Part model, mm, in its own coordinate system. A direction names the side the tool comes from. Round coordinates to 2 decimals unless told otherwise and drop trailing zeros. Order: outer loops, then holes, each group sorted by start corner. A loop starts at its lowest first (then second) coordinate and runs counter-clockwise, first axis right, second up. Notation, with made-up numbers: (-34.5, 41.5) - (-27.5, 41.5) arc R26 ccw to (-27.5, 66.5) - close; hole circle Ø3 at (64.5, -3.5). An arc over 180 degrees is marked (long way). Answer as a JSON object with one key per item and string values.
```python
from build123d import *

# Parameters (mm, degrees)
RESSALTO_EXTRUS_O1_DEPTH = 6
ESBO_O2_R                = 3.55
RESSALTO_EXTRUS_O2_DEPTH = 2.45
CORTE_EXTRUS_O1_DEPTH    = 12.406502719
CORTE_EXTRUS_O2_REACH    = 13.407
ESBO_O4_R                = 2.525
CHANFRO2_SIZE            = 0.25
CHANFRO3_SIZE            = 0.1


with BuildPart() as part:
    # Esboço1 → Ressalto-extrusão1 (new body)
    with BuildSketch(Plane.XY):
        Polygon((4.961441577, -2.952529562), (5.037686394, 2.820469664), (0.076244817, 5.772999226), (-4.961441577, 2.952529562), (-5.037686394, -2.820469664), (-0.076244817, -5.772999226), align=None)
    extrude(amount=RESSALTO_EXTRUS_O1_DEPTH)

    # Esboço2 → Ressalto-extrusão2 (add)
    with BuildSketch(Plane.XY.offset(6)):
        Circle(ESBO_O2_R)
    extrude(amount=RESSALTO_EXTRUS_O2_DEPTH)

    # Esboço3 → Corte-extrusão1 (cut, through all)
    with BuildSketch(Plane(origin=(0, 0, 0), x_dir=(-1, 0, 0), z_dir=(0, 0, -1))):
        Polygon((-1.65800996, 4.831698543), (-2.173420765, 3.652224278), (-3.376703738, 3.808912301), align=None)
    extrude(amount=-CORTE_EXTRUS_O1_DEPTH, mode=Mode.SUBTRACT)

    # Esboço4 → Corte-extrusão2 (cut, up to next)
    with BuildSketch(Plane.XY.offset(8.45), mode=Mode.PRIVATE) as corte_extrus_o2_sk1:
        with Locations((0, 0.375)):
            Circle(ESBO_O4_R)
    corte_extrus_o2_tool1 = extrude(corte_extrus_o2_sk1.sketch, amount=-CORTE_EXTRUS_O2_REACH, mode=Mode.PRIVATE) & part.part
    add(corte_extrus_o2_tool1.solids().sort_by_distance((0, 0.375, 8.45))[0], mode=Mode.SUBTRACT)

    # Chanfro2
    chanfro2_edges = [part.edges().sort_by_distance(p)[0] for p in [
        (4.999563986, -0.066029949, 0),
        (2.44259838, -4.362764394, 0),
        (4.207195066, 3.314690983, 0),
        (-2.556965606, -4.296734445, 0),
        (-4.999563986, 0.066029949, 0),
        (-2.44259838, 4.362764394, 0),
        (2.775062251, 3.73056829, 0),
        (0.867127389, 5.302348884, 0),
        (1.915715362, 4.241961411, 0),
        (-2.525, 0.375, 0),
    ]]
    chamfer(chanfro2_edges, length=CHANFRO2_SIZE)

    # Chanfro3
    chanfro3_edges = [part.edges().sort_by_distance(p)[0] for p in [
        (-3.55, 0, 8.45),
        (-2.525, 0.375, 8.45),
    ]]
    chamfer(chanfro3_edges, length=CHANFRO3_SIZE)


solid = part.part
```
Item 1: Tool access for faces 4 (the flat face through (0, -4, 6)), 5 (the flat face through (-2.592, -4.276, 3.085)), 6 (the flat face through (2.77, 3.73, 3.08)): list every direction of +Z, -Z, +X, -X, +Y, -Y with a clear straight run to the whole face (end or side of a thin tool).
Taken from the geometry:
{"face 4": "+Z", "face 5": "+Z, -Z, -X, -Y", "face 6": "+Z, -Z, +Y"}
Item 2: Cut at C-C (z = 6.5). Write the cut outline in (x, y) (3 decimals), plus the area to 3 significant figures.
Taken from the geometry:
{"outline": "circle Ø7.1 at (0, 0); hole circle Ø5.05 at (0, 0.375)", "area": "19.6 mm2"}
Item 3: Cut at A-A (z = 2). Write the cut outline in (x, y) (3 decimals).
Taken from the geometry:
{"outline": "(-5.038, -2.82) - (-0.076, -5.773) - (4.961, -2.953) - (5.038, 2.82) - (3.377, 3.809) - (2.173, 3.652) - (1.658, 4.832) - (0.076, 5.773) - (-4.961, 2.953) - close; hole circle Ø5.05 at (0, 0.375)"}
Item 4: Drop flat-ended pins along their axis: P1, Ø1.5, axis at x = 3.5, y = 0.5, coming from the +Z side; P2, Ø4, axis at x = -2.5, z = 5, coming from the -Y side; P3, Ø4, axis at y = 0, z = 5, coming from the -X side; P4, Ø2, axis at x = -2, z = 5, coming from the +Y side. Give the stop position or say it passes through.
Taken from the geometry:
{"P1": "z = 8.45", "P2": "y = -5.52", "P3": "x = -5.03", "P4": "y = 5.17"}
Item 5: Two-plate mould, pull along Y, no slides. Class faces 1 (the cylindrical face through (2.41, 1.13, 4.36)), 2 (the flat face through (4.15, 3.2, 0.12)), 3 (the cylindrical face through (-0.46, 3.52, 7.16)): pulls with the +Y half, pulls with the -Y half, needs draft (parallel to the pull), parting line crosses it, or undercut.
Taken from the geometry:
{"face 1": "undercut", "face 2": "pulls with the +Y half", "face 3": "parting line crosses it"}
Item 6: Cut at B-B (x = 4.25). Write the cut outline in (y, z).
Taken from the geometry:
{"outline": "(-3.35, 0.25) - (-3.06, 0) - (3, 0) - (3.29, 0.25) - (3.29, 6) - (-3.35, 6) - close"}
Item 7: Probe L1, parallel to Z at x = -4.5, y = -1; L2, parallel to Y at x = 0, z = 5.75; L3, parallel to X at y = 2.5, z = 3.75. List the from-to ranges inside material, lowest first. Write a range as from..to.
Taken from the geometry:
{"L1": "0..6", "L2": "-5.73..-2.15, 2.9..5.73", "L3": "-4.97..-1.36, 1.36..5.03"}
